```python
from build123d import *

# Parameters (mm, degrees)
EXTRUDE_1_DEPTH     = 400
SKETCH_2_R          = 3.25
CUT_EXTRUDE_1_DEPTH = 5.3
SKETCH_3_R          = 2.25
CUT_EXTRUDE_2_DEPTH = 10.7


with BuildPart() as part:
    # Model → Бобышка-Вытянуть1 (new body)
    with BuildSketch(Plane.XY):
        with BuildLine():
            Line((6.8, 0), (7.5, 0.7))
            Line((7.5, 0.7), (7.5, 3.6994391))
            Line((7.5, 3.6994391), (4.7998047, 6.3996344))
            Line((4.7998047, 6.3996344), (4.7998047, 8.409149262))
            Line((4.7998047, 8.409149262), (5.20075838, 8.810103152))
            ThreePointArc((5.20075838, 8.810103152), (5.668922208, 9.789261508), (6.648080611, 10.257425237))
            Line((6.648080611, 10.257425237), (7.5, 11.109345046))
            Line((7.5, 11.109345046), (7.5, 12.449454443))
            Line((7.5, 12.449454443), (6.634490912, 13.314965186))
            ThreePointArc((6.634490912, 13.314965186), (5.668922174, 13.781617126), (5.202270193, 14.747185846))
            Line((5.202270193, 14.747185846), (4.949456226, 15))
            Line((4.949456226, 15), (-4.949456226, 15))
            Line((-4.949456226, 15), (-5.202270193, 14.747185846))
            ThreePointArc((-5.202270193, 14.747185846), (-5.668922174, 13.781617126), (-6.634490912, 13.314965186))
            Line((-6.634490912, 13.314965186), (-7.5, 12.449454443))
            Line((-7.5, 12.449454443), (-7.5, 11.109345046))
            Line((-7.5, 11.109345046), (-6.648080611, 10.257425238))
            ThreePointArc((-6.648080611, 10.257425238), (-5.668922208, 9.789261508), (-5.20075838, 8.810103152))
            Line((-5.20075838, 8.810103152), (-4.7998047, 8.409149262))
            Line((-4.7998047, 8.409149262), (-4.7998047, 6.3996344))
            Line((-4.7998047, 6.3996344), (-7.5, 3.6994391))
            Line((-7.5, 3.6994391), (-7.5, 0.7))
            Line((-7.5, 0.7), (-6.8, 0))
            Line((-6.8, 0), (6.8, 0))
        make_face()
    extrude(amount=EXTRUDE_1_DEPTH)

    # Эскиз2 → Вырез-Вытянуть1 (cut)
    with BuildSketch(Plane(origin=(0, 15, 0), x_dir=(1, 0, 0), z_dir=(0, 1, 0))):
        with Locations((0, -30)):
            Circle(SKETCH_2_R)
        with Locations((0, -90)):
            Circle(SKETCH_2_R)
        with Locations((0, -150)):
            Circle(SKETCH_2_R)
        with Locations((0, -210)):
            Circle(SKETCH_2_R)
        with Locations((0, -270)):
            Circle(SKETCH_2_R)
        with Locations((0, -330)):
            Circle(SKETCH_2_R)
        with Locations((0, -390)):
            Circle(SKETCH_2_R)
        with Locations((0, -450)):
            Circle(SKETCH_2_R)
        with Locations((0, -510)):
            Circle(SKETCH_2_R)
        with Locations((0, -570)):
            Circle(SKETCH_2_R)
    extrude(amount=-CUT_EXTRUDE_1_DEPTH, mode=Mode.SUBTRACT)

    # Эскиз3 → Вырез-Вытянуть2 (cut, through all)
    with BuildSketch(Plane(origin=(0, 9.7, 0), x_dir=(1, 0, 0), z_dir=(0, 1, 0))):
        with Locations((0, -30)):
            Circle(SKETCH_3_R)
        with Locations((0, -90)):
            Circle(SKETCH_3_R)
        with Locations((0, -150)):
            Circle(SKETCH_3_R)
        with Locations((0, -210)):
            Circle(SKETCH_3_R)
        with Locations((0, -270)):
            Circle(SKETCH_3_R)
        with Locations((0, -330)):
            Circle(SKETCH_3_R)
        with Locations((0, -390)):
            Circle(SKETCH_3_R)
        with Locations((0, -450)):
            Circle(SKETCH_3_R)
        with Locations((0, -510)):
            Circle(SKETCH_3_R)
        with Locations((0, -570)):
            Circle(SKETCH_3_R)
    extrude(amount=-CUT_EXTRUDE_2_DEPTH, mode=Mode.SUBTRACT)


solid = part.part
```
Model file for the job. Use its own axes, mm. A direction names the side the tool comes from. Round coordinates to 2 decimals unless told otherwise and drop trailing zeros. Write each loop counter-clockwise with the first axis right and the second up, starting at its lowest first coordinate (ties: lowest second). Pieces come first, ordered by that corner, then holes. Notation, with made-up numbers: M 2.5,78 L 24.5,78 A9 cw 24.5,87 Z; hole C 51,-1 d1. An arc over 180 degrees is marked long. Put each result on its own line as item: value.
Item 1: Cut at B-B (x = 0). State how many separate pieces and enclosed holes the cut face has, and give its area (3 significant figures).
Responses:
separate pieces: 8
enclosed holes: 0
area: 5,450 mm²
Item 2: Probe L1, parallel to X at y = 7, z = 390; L2, parallel to X at y = 6.25, z = 90; L3, parallel to X at y = 6.5, z = 255.5. List the from-to ranges inside material, lowest first. Write a range as from..to.
Responses:
L1: -4.8..-2.25, 2.25..4.8
L2: -4.95..-2.25, 2.25..4.95
L3: -4.8..4.8
Item 3: Flat gauge pins, fed straight in: P1, Ø6, axis at x = 0, z = 150, coming from the +Y side; P2, Ø3.5, axis at x = 0, z = 210, coming from the -Y side. Where does each tip first touch, or does it go through?
Responses:
P1: y = 9.7
P2: through
Item 4: Cut at A-A (z = 78). List the corners of the cut face in (x, y), and give its area (3 significant figures).
Responses:
outline: M -7.5,0.7 L -6.8,0 L 6.8,0 L 7.5,0.7 L 7.5,3.7 L 4.8,6.4 L 4.8,8.41 L 5.2,8.81 A1.63 cw 6.65,10.26 L 7.5,11.11 L 7.5,12.45 L 6.63,13.31 A1.63 cw 5.2,14.75 L 4.95,15 L -4.95,15 L -5.2,14.75 A1.63 cw -6.63,13.31 L -7.5,12.45 L -7.5,11.11 L -6.65,10.26 A1.63 cw -5.2,8.81 L -4.8,8.41 L -4.8,6.4 L -7.5,3.7 Z
area: 191 mm²
Item 5: Tool access for faces 1 (the flat face through (0, 15, 197)), 2 (the cylindrical face through (-0.705, 12.387, 393.173)): list every direction of +Z, -Z, +X, -X, +Y, -Y with a clear straight run to the whole face (end or side of a thin tool).
Responses:
face 1: +Z, -Z, +X, -X, +Y
face 2: +Y
